Input: part model. Units: mm. Frame: model coordinates. Face numbers are marked on the shaded views. A direction names the side the tool comes from. Give positions to 0.01 mm unless a question says otherwise; leave off trailing zeros. Loops run counter-clockwise (first coordinate to the right, second up) from the corner with the lowest first, then second, coordinate; pieces in that order, holes last. Notation, with made-up numbers: (58.5, 39) - (77.5, 39) arc R18 cw to (77.5, 72) - close; hole circle Ø11 at (27.25, -32). An arc over 180 degrees is marked (long way). Answer as a JSON object with one key per item and string values. Group by question number.
(1) Section query C-C (y = 76). Return loops of the section in (x, z).
(2) Mould query, pull axis Z, two halves, no side actions, for the marked faces 5, 6 and 7. Classes: +Z half, -Z half, draft (parallel to the pull), parting line (faces both ways), or undercut.
(3) Access query for the marked faces 1, 2, 3 and 4. Directions: +Z, -Z, +X, -X, +Y, -Y. A direction counts if a zero-diameter tool reaches every point of the face in a straight line with its end or side. Return the directions, or none.
(4) Section query A-A (x = 118.5). Return loops of the section in (y, z), plus the area to 3 significant figures.
(5) Section query D-D (z = -291.5). Return loops of the section in (x, y).
(6) Material intervals for L1, parallel to Z at x = 304, y = 72; L2, parallel to X at y = 173, z = -33; L3, parallel to X at y = 68, z = -144, sorted ascending.
(7) Pin query (flat end, axial travel): P1, Ø5, axis at y = 236.5, z = -258, coming from the -X side; P2, Ø3, axis at y = 71.5, z = -220, coming from the +X side; P3, Ø4.5, axis at x = 313.5, z = -202.5, coming from the -Y side. Return the tip coordinate at first contact, or that it passes through.
(8) Section query B-B (z = -103). Return loops of the section in (x, y).
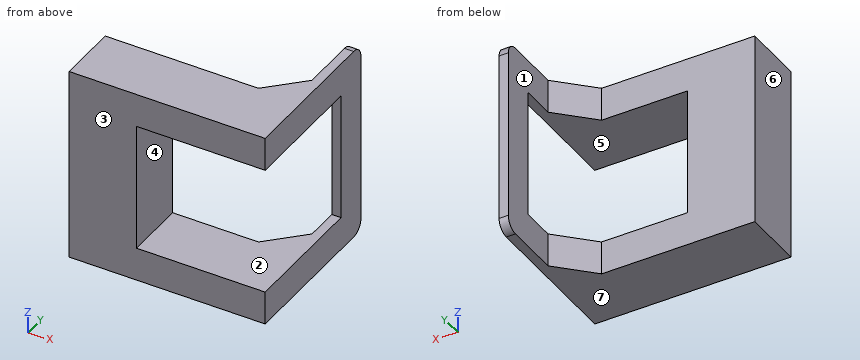
```python
from build123d import *

# Parameters (mm, degrees)
EXTRUDE_1_DEPTH = 100
EXTRUDE_2_DEPTH = 15
EXTRUDE_3_DEPTH = 55
EXTRUDE_4_DEPTH = 55
FILLET_1_R      = 20


with BuildPart() as part:
    # 草图1 → 凸台-拉伸1 (new body)
    with BuildSketch(Plane(origin=(0, 0, 0), x_dir=(1, 0, 0), z_dir=(0, 1, 0))):
        Polygon((0, 0), (320, 0), (320, 55), (110, 55), (110, 265), (320, 265), (320, 320), (0, 320), align=None)
    extrude(amount=EXTRUDE_1_DEPTH)

    # 草图2 → 凸台-拉伸2 (add)
    with BuildSketch(Plane(origin=(320, 0, 0), x_dir=(0, 0, -1), z_dir=(1, 0, 0))):
        Polygon((0, 0), (0, 265), (320, 265), (320, 0), (265, 0), (265, 210), (55, 210), (55, 0), align=None)
    extrude(amount=-EXTRUDE_2_DEPTH)

    # 草图3 → 凸台-拉伸3 (add)
    with BuildSketch(Plane.XY):
        Polygon((250, 100), (305, 100), (305, 155), align=None)
    extrude(amount=-EXTRUDE_3_DEPTH)

    # 草图4 → 凸台-拉伸4 (add)
    with BuildSketch(Plane(origin=(0, 0, -320), x_dir=(-1, 0, 0), z_dir=(0, 0, -1))):
        Polygon((-305, 155), (-305, 100), (-250, 100), align=None)
    extrude(amount=-EXTRUDE_4_DEPTH)

    # 圆角1
    fillet_1_edges = [part.edges().sort_by_distance(p)[0] for p in [
        (312.5, 265, -320),
        (312.5, 265, 0),
    ]]
    fillet(fillet_1_edges, radius=FILLET_1_R)


solid = part.part
```
Recorded:
{
 "1": {"outline": "(0, -320) - (320, -320) - (320, -265) - (110, -265) - (110, -55) - (320, -55) - (320, 0) - (0, 0) - close"},
 "2": {"face 5": "undercut", "face 6": "draft", "face 7": "-Z half"},
 "3": {"face 1": "+Z, -Z, -X, +Y", "face 2": "+X, -Y", "face 3": "+Z, -Z, +X, -X, -Y", "face 4": "+X, +Y, -Y"},
 "4": {"outline": "(0, -320) - (100, -320) - (100, -265) - (0, -265) - close; (0, -55) - (100, -55) - (100, 0) - (0, 0) - close", "area": "11,000 mm^2"},
 "5": {"outline": "(0, 0) - (320, 0) - (320, 265) - (305, 265) - (305, 155) - (250, 100) - (0, 100) - close"},
 "6": {"L1": "z = -320 to -265, -55 to 0", "L2": "x = 305 to 320", "L3": "x = 0 to 110"},
 "7": {"P1": "stops at x = 305", "P2": "stops at x = 110", "P3": "stops at y = 210"},
 "8": {"outline": "(0, 0) - (110, 0) - (110, 100) - (0, 100) - close; (305, 210) - (320, 210) - (320, 265) - (305, 265) - close"}
}
